from build123d import *

# Parameters (mm, degrees)
F1_DEPTH  = 20
F0_W      = 1.5
F0_H      = 45.8000004292
F0_W_2    = 46.8000004292
F0_H_2    = 1.5
F2_DEPTH  = 5
F3_R      = 5
F5_DEPTH  = 150.7
F7_DEPTH  = 137.6
F13_DEPTH = 60
F14_DEPTH = 56.1
F20_DEPTH = 72.8
F21_DEPTH = 71.7


with BuildPart() as f1:
    # F0 (on Top) → F1 (new body)
    with BuildSketch(Plane.XY):
        with BuildLine():
            Line((37, 63.7), (-37, 63.7))
            ThreePointArc((-37, 63.7), (-55.5261976671, 56.0261976671), (-63.2, 37.5))
            Line((-63.2, 37.5), (-63.2, -37.5))
            ThreePointArc((-63.2, -37.5), (-55.5261976671, -56.0261976671), (-37, -63.7))
            Line((-37, -63.7), (37, -63.7))
            ThreePointArc((37, -63.7), (55.5261976671, -56.0261976671), (63.2, -37.5))
            Line((63.2, -37.5), (63.2, 37.5))
            ThreePointArc((63.2, 37.5), (55.5261976671, 56.0261976671), (37, 63.7))
        make_face()
        with BuildLine():
            ThreePointArc((-62, 37.5), (-54.6776695297, 55.1776695297), (-37, 62.5))
            Line((-37, 62.5), (-2.5, 62.5))
            Line((-2.5, 62.5), (-1, 62.5))
            Line((-1, 62.5), (1, 62.5))
            Line((1, 62.5), (2.5, 62.5))
            Line((2.5, 62.5), (37, 62.5))
            ThreePointArc((37, 62.5), (54.6776695297, 55.1776695297), (62, 37.5))
            Line((62, 37.5), (62, 1.5))
            Line((62, 1.5), (62, 0))
            Line((62, 0), (62, -1.5))
            Line((62, -1.5), (62, -3))
            Line((62, -3), (62, -37.5))
            ThreePointArc((62, -37.5), (54.6776695297, -55.1776695297), (37, -62.5))
            Line((37, -62.5), (-37, -62.5))
            ThreePointArc((-37, -62.5), (-54.6776695297, -55.1776695297), (-62, -37.5))
            Line((-62, -37.5), (-62, -3))
            Line((-62, -3), (-62, -1.5))
            Line((-62, -1.5), (-62, 0))
            Line((-62, 0), (-62, 1.5))
            Line((-62, 1.5), (-62, 37.5))
        make_face(mode=Mode.SUBTRACT)
    extrude(amount=F1_DEPTH)

    # F0 (on Top) → F2 (join)
    with BuildSketch(Plane.XY):
        with Locations((1.75, 39.5999997854)):
            Rectangle(F0_W, F0_H)
        Polygon((-1, 16.6999995708), (-2.5, 16.6999995708), (-15.1999995708, 16.6999995708), (-15.1999995708, 1.5), (-15.1999995708, 0), (-15.1999995708, -1.5), (-15.1999995708, -3), (-15.1999995708, -16.6999995708), (-15.1999995708, -20), (-13.5, -20), (-13.5, -15), (-13.5, 15), (13.5, 15), (13.5, -15), (13.5, -20), (15.1999995708, -20), (15.1999995708, -15), (15.1999995708, -3), (15.1999995708, -1.5), (15.1999995708, 0), (15.1999995708, 1.5), (15.1999995708, 16.6999995708), (2.5, 16.6999995708), (1, 16.6999995708), align=None)
        with Locations((-1.75, 39.5999997854)):
            Rectangle(F0_W, F0_H)
        with Locations((-38.5999997854, 0.75)):
            Rectangle(F0_W_2, F0_H_2)
        with Locations((-38.5999997854, -2.25)):
            Rectangle(F0_W_2, F0_H_2)
        with Locations((38.5999997854, 0.75)):
            Rectangle(F0_W_2, F0_H_2)
        with Locations((38.5999997854, -2.25)):
            Rectangle(F0_W_2, F0_H_2)
    extrude(amount=F2_DEPTH)

    # F3
    f3_edges = [f1.edges().sort_by_distance(p)[0] for p in [
        (-2.5, 62.5, 2.5),
        (2.5, 62.5, 2.5),
        (-2.5, 16.7, 2.5),
        (2.5, 16.7, 2.5),
        (62, 1.5, 2.5),
        (15.2, 1.5, 2.5),
        (62, -3, 2.5),
        (15.2, -3, 2.5),
        (-15.2, -3, 2.5),
        (-62, -3, 2.5),
        (-62, 1.5, 2.5),
        (-15.2, 1.5, 2.5),
        (1.75, 62.5, 5),
        (-1.75, 62.5, 5),
        (62, 0.75, 5),
        (62, -2.25, 5),
        (-62, 0.75, 5),
        (-62, -2.25, 5),
    ]]
    fillet(f3_edges, radius=F3_R)

    # F4 (on face) → F5 (cut)
    with BuildSketch(Plane(origin=(0, 63.7, 0), x_dir=(-1, 0, 0), z_dir=(0, 1, 0))):
        Polygon((37, 20), (-37, 20), (-25.8996840566, 12.3994192109), (0, 10.6452321634), (25.8996840566, 12.3994192109), align=None)
    extrude(amount=-F5_DEPTH, mode=Mode.SUBTRACT)

    # F6 (on face) → F7 (cut)
    with BuildSketch(Plane(origin=(-63.2, 0, 0), x_dir=(0, -1, 0), z_dir=(-1, 0, 0))):
        Polygon((37.5, 20), (-37.5, 20), (-26.3996840566, 12.3994192109), (0, 10.6842042878), (26.3996840566, 12.3994192109), align=None)
    extrude(amount=-F7_DEPTH, mode=Mode.SUBTRACT)

    # F12 (on face) → F13 (cut)
    with BuildSketch(Plane(origin=(-74.2462120246, -74.2462120246, 0), x_dir=(-0.7071067812, 0.7071067812, 0), z_dir=(0.7071067812, 0.7071067812, 0))):
        Polygon((-12, 10), (-38.037519902, 0), (38.037519902, 0), (12, 10), (0, 10), align=None)
    extrude(amount=F13_DEPTH, mode=Mode.SUBTRACT)

    # F10 (on face) → F14 (cut)
    with BuildSketch(Plane(origin=(71.6299169342, 71.6299169342, 0), x_dir=(-0.7071067812, 0.7071067812, 0), z_dir=(0.7071067812, 0.7071067812, 0))):
        Polygon((-38.037519902, 0), (0, 0), (0, 10), (-12, 10), align=None)
        Polygon((0, 10), (0, 0), (38.037519902, 0), (12, 10), align=None)
    extrude(amount=-F14_DEPTH, mode=Mode.SUBTRACT)

    # F19 (on face) → F20 (cut)
    with BuildSketch(Plane(origin=(84.1457069612, -84.1457069612, 0), x_dir=(-0.7071067812, -0.7071067812, 0), z_dir=(-0.7071067812, 0.7071067812, 0))):
        Polygon((-12.000480098, 10), (-38.038, 0), (38.037039804, 0), (11.999519902, 10), (-0.000480098, 10), align=None)
    extrude(amount=F20_DEPTH, mode=Mode.SUBTRACT)

    # F18 (on face) → F21 (cut)
    with BuildSketch(Plane(origin=(-82.0243866176, 82.0243866176, 0), x_dir=(-0.7071067812, -0.7071067812, 0), z_dir=(-0.7071067812, 0.7071067812, 0))):
        Polygon((-12.000480098, 10), (-38.038, 0), (38.037039804, 0), (11.999519902, 10), (-0.000480098, 10), align=None)
    extrude(amount=-F21_DEPTH, mode=Mode.SUBTRACT)


solid = f1.part
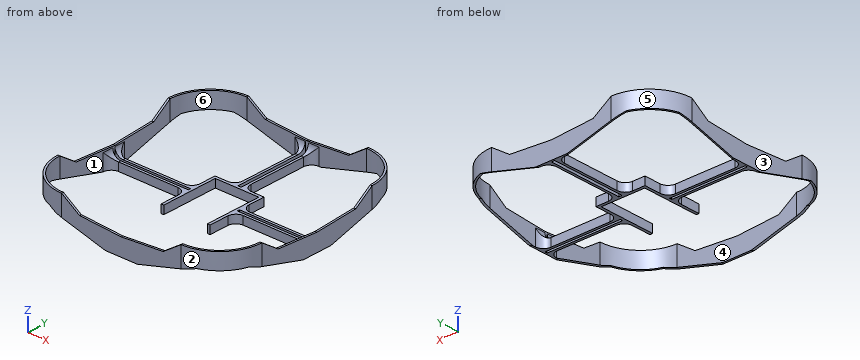
Geometry: final body of the model. Coordinates: model frame, mm. Face numbers are marked on the shaded views. A direction names the side the tool comes from. Round coordinates to 2 decimals unless told otherwise and drop trailing zeros. Loops run counter-clockwise (first coordinate to the right, second up) from the corner with the lowest first, then second, coordinate; pieces in that order, holes last.
Q1. Section B-B on x = -28.5. Return loops of the section in (y, z).
Q2. Section D-D on y = -52. Return loops of the section in (x, z).
Q3. Access query for the marked faces 5 and 6. Directions: +Z, -Z, +X, -X, +Y, -Y. A direction counts if a zero-diameter tool reaches every point of the face in a straight line with its end or side. Return the directions, or none.
Q4. Section C-C on z = 17.5. State how many separate pieces and enclosed holes the cut face has, plus the area to 3 significant figures.
Q5. Pin query (flat end, axial travel): P1, Ø4, axis at x = 41.5, z = 3.5, coming from the -Y side; P2, Ø3, axis at y = 36.5, z = 4.5, coming from the -X side; P3, Ø23, axis at x = 19, y = 13.5, coming from the +Z side. Return the tip coordinate at first contact, or that it passes through.
Q6. Section A-A on y = -13. Return loops of the section in (x, z), plus the area to 3 significant figures.
Q7. Pull-direction query (X, two-part tool) for the marked faces 1, 2, 3 and 4; classes: released by +X, released by -X, zero draft, split by the parting line, or undercut.
Q8. Material intervals for L1, parallel to Y at x = 52, z = 3.75; L2, parallel to X at y = 21, z = 10.75; L3, parallel to Y at x = -27.5, z = 10, sorted ascending.
Evaluation:
1. outline: (-63.7, 5.05) - (-62.5, 5.38) - (-62.5, 14.18) - (-63.7, 14.18) - close; (-3, 0) - (-1.5, 0) - (-1.5, 5) - (-3, 5) - close; (0, 0) - (1.5, 0) - (1.5, 5) - (0, 5) - close; (62.5, 5.38) - (63.7, 5.05) - (63.7, 14.18) - (62.5, 14.18) - close
2. outline: (-58.82, 10) - (-57.37, 10) - (-57.37, 20) - (-58.82, 20) - close; (57.37, 10) - (58.82, 10) - (58.82, 20) - (57.37, 20) - close
3. face 5: +Z, -Z, -X, +Y
3. face 6: +Z, -Z
4. separate pieces: 4
4. enclosed holes: 0
4. area: 228 mm2
5. P1: stops at y = -3
5. P2: stops at x = -2.5
5. P3: stops at z = 5
6. outline: (-63.2, 0.98) - (-62, 1.3) - (-62, 11.53) - (-63.2, 11.53) - close; (-15.2, 0) - (-13.5, 0) - (-13.5, 5) - (-15.2, 5) - close; (13.5, 0) - (15.2, 0) - (15.2, 5) - (13.5, 5) - close; (62, 1.3) - (63.2, 0.98) - (63.2, 11.53) - (62, 11.53) - close
6. area: 41.9 mm2
7. face 1: undercut
7. face 2: released by +X
7. face 3: released by -X
7. face 4: undercut
8. L1: y = -3 to -1.5, 0 to 1.5
8. L2: x = -63.2 to -62, 62 to 63.2
8. L3: y = -63.7 to -62.5, 62.5 to 63.7
